Input: part model. Units: mm. Frame: model coordinates. Give positions to 0.01 mm unless a question says otherwise; leave off trailing zeros. Write each loop counter-clockwise with the first axis right and the second up, starting at its lowest first coordinate (ties: lowest second). Pieces come first, ordered by that corner, then holes.
```python
from build123d import *

# Parameters (mm, degrees)
F0_W     = 40
F0_H     = 25
F1_DEPTH = 3
F4_D     = 5
F5_R     = 1


with BuildPart() as f1:
    # F0 (on Top) → F1 (new body)
    with BuildSketch(Plane.XY):
        with Locations((0, 32.112984)):
            Rectangle(F0_W, F0_H)
    extrude(amount=F1_DEPTH)

    # F4 (through all)
    with Locations(Plane.XY.offset(5)):
        with Locations((-12.205, 32.112984), (12.205, 32.112984)):
            Hole(F4_D / 2)

    # F5
    f5_edges = [f1.edges().sort_by_distance(p)[0] for p in [
        (0, 44.612984, 3),
        (20, 32.112984, 3),
        (-20, 32.112984, 3),
        (0, 19.612984, 3),
        (-14.705, 32.112984, 3),
        (9.705, 32.112984, 3),
    ]]
    fillet(f5_edges, radius=F5_R)


solid = f1.part
```
Item 1: Pin query (flat end, axial travel): pin 1 (3 mm diameter, centred on x = -12.2, y = 32.11, fed in from -Z). Return the tip coordinate at first contact, or that it passes through.
Item 2: Section A-A (z = 2.45). Return loops of the section in (x, y) (3 decimals).
Item 3: Ray query, line 1 (X direction, y = 33.75, z = 1.5); line 2 (X direction, y = 32.75, z = 2.4); line 3 (Y direction, x = -12, z = 0.55). Return the intervals inside material, ascending.
Item 4: Section B-B (y = 32.5). Give the number of separate pieces and of enclosed holes in the cut face, and give its area (3 significant figures).
Item 5: Mould query, pull axis Y, two halves, no side actions, for faces 1 (the flat face through (0, 32, 0)), 2 (the cylindrical face through (-13.359, 29.895, 0.986)), 3 (the cylindrical face through (0.3, 19.9, 2.7)). Classes: +Y half, -Y half, draft (parallel to the pull), parting line (faces both ways), or undercut.
Solved:
1. pin 1: passes through
2. outline: (-19.893, 19.72) - (19.893, 19.72) - (19.893, 44.506) - (-19.893, 44.506) - close; hole circle Ø5.214 at (-12.205, 32.113); hole circle Ø5.214 at (12.205, 32.113)
3. line 1: x = -20 to -14.09, -10.32 to 10.32, 14.09 to 20
3. line 2: x = -19.92 to -14.71, -9.7 to 9.7, 14.71 to 19.92
3. line 3: y = 19.61 to 29.62, 34.6 to 44.61
4. separate pieces: 3
4. enclosed holes: 0
4. area: 89.1 mm2
5. face 1: draft
5. face 2: undercut
5. face 3: -Y half
